Build history of the part. All positions in model axes, mm. A direction names the side the tool comes from. Round coordinates to 2 decimals unless told otherwise and drop trailing zeros. Order: outer loops, then holes, each group sorted by start corner. A loop starts at its lowest first (then second) coordinate and runs counter-clockwise, first axis right, second up. Notation, with made-up numbers: (19, 15.5) -> (53, 15.5) arc R19 cw to (53, 47.5) -> close; hole circle Ø4 at (50, 6). An arc over 180 degrees is marked (long way). Use a Markdown table: item, result. Add a question column.
Item 1: Pin check, flat tips, straight feed: pin 1 (1 mm diameter, centred on x = 31, z = 1, fed in from -Y); pin 2 (0.7 mm diameter, centred on x = 33.5, z = 1.5, fed in from -Y); pin 3 (0.8 mm diameter, centred on y = -18, z = 1.5, fed in from +X). Stop position of each tip, or through.
Item 2: Slice it at A-A, the plane y = -15. Give the cut face in (x, z).
Item 3: 3-axis set-ups, long thin cutter, end or side, ignore diameter. For faces 5 (the face through (15.894, -8, 1)), 6 (the face through (34, -13.45, 1)): which of +Z, -Z, +X, -X, +Y, -Y reach the whole face in a straight line?
Item 4: Slice it at D-D, the plane x = 32.75. Give the cut face in (y, z).
Item 5: Probe L1, parallel to X at y = -8.5, z = 0.95; L2, parallel to Y at x = 27, z = 0.5; L3, parallel to Y at x = 28.25, z = 0.45. List the from-to ranges inside material, lowest first.
Item 6: Slice it at B-B, the plane z = 1.7. Give the cut face in (x, y), plus the area to 3 significant figures.
Item 7: Two-plate mould, pull along X, no slides. Class faces 1 (the face through (25, -6, 2.286)), 2 (the face through (26.05, -8.79, 1.13)), 3 (the face through (28.95, -15.75, 1.13)), 4 (the face through (34.175, -6, 1)): released by +X, released by -X, zero draft, split by the parting line, or undercut.
Item 8: Slice it at C-C, the plane y = -10.5. Give the cut face in (x, z).
from build123d import *

# Parameters (mm, degrees)
F0_R     = 2.032
F1_DEPTH = 2.286


with BuildPart() as f1:
    # F0 (on Top) → F1 (new body)
    with BuildSketch(Plane.XY):
        with BuildLine():
            Line((34.175198, -8.878299), (34.175198, 2.043701))
            Line((34.175198, 2.043701), (15.893778, 2.043701))
            Line((15.893778, 2.043701), (15.893778, -13.450299))
            Line((15.893778, -13.450299), (15.893778, -18.530299))
            Line((15.893778, -18.530299), (19.703778, -18.530299))
            Line((19.703778, -18.530299), (19.703778, -17.006299))
            ThreePointArc((19.703778, -17.006299), (21.185336, -14.485536), (24.108456, -14.553586))
            ThreePointArc((24.108456, -14.553586), (24.203978, -14.6154), (24.296988, -14.680933))
            ThreePointArc((24.296988, -14.680933), (29.019072, -15.740683), (33.282321, -13.450299))
            Line((33.282321, -13.450299), (34.175198, -13.450299))
            Line((34.175198, -13.450299), (34.175198, -8.878299))
        make_face()
        with Locations((28.079198, -8.878299)):
            Circle(F0_R, mode=Mode.SUBTRACT)
    extrude(amount=F1_DEPTH)


solid = f1.part
Check sheet entries:
| question | item | result |
|---|---|---|
| 1 | pin 1 | y = -15.37 |
| 1 | pin 2 | y = -13.6 |
| 1 | pin 3 | x = 19.7 |
| 2 | outline | (15.89, 0) -> (20.52, 0) -> (20.52, 2.29) -> (15.89, 2.29) -> close; (24.84, 0) -> (31.32, 0) -> (31.32, 2.29) -> (24.84, 2.29) -> close |
| 3 | face 5 | +Z, -Z, -X, +Y, -Y |
| 3 | face 6 | +Z, -Z, +X, -Y |
| 4 | outline | (-13.99, 0) -> (2.04, 0) -> (2.04, 2.29) -> (-13.99, 2.29) -> close |
| 5 | L1 | 15.89 to 26.08, 30.08 to 34.18 |
| 5 | L2 | -15.72 to -10.6, -7.16 to 2.04 |
| 5 | L3 | -15.8 to -10.9, -6.85 to 2.04 |
| 6 | outline | (15.89, -18.53) -> (19.7, -18.53) -> (19.7, -17.01) arc R2.89 cw to (24.11, -14.55) arc R2.88 cw to (24.3, -14.68) arc R6.93 ccw to (33.28, -13.45) -> (34.18, -13.45) -> (34.18, 2.04) -> (15.89, 2.04) -> close; hole circle Ø4.06 at (28.08, -8.88) |
| 6 | area | 311 mm2 |
| 7 | face 1 | zero draft |
| 7 | face 2 | undercut |
| 7 | face 3 | undercut |
| 7 | face 4 | released by +X |
| 8 | outline | (15.89, 0) -> (26.85, 0) -> (26.85, 2.29) -> (15.89, 2.29) -> close; (29.3, 0) -> (34.18, 0) -> (34.18, 2.29) -> (29.3, 2.29) -> close |
